CAD build for the part. Positions are in the model's coordinates, mm. A direction names the side the tool comes from. Coordinates: 2 decimals unless noted, no trailing zeros. Loops run counter-clockwise (first coordinate to the right, second up) from the corner with the lowest first, then second, coordinate; pieces in that order, holes last. Notation, with made-up numbers: (71, 69) - (103, 69) arc R24 ccw to (103, 99) - close; hole circle Ø6 at (87.5, 35.5). An arc over 180 degrees is marked (long way). Put each result on its own line as item: value.
```python
from build123d import *

# Parameters (mm, degrees)
SKETCH_1_W          = 28
SKETCH_1_H          = 45
EXTRUDE_1_DEPTH     = 2
SKETCH_2_W          = 25.5
SKETCH_2_H          = 40
EXTRUDE_2_DEPTH     = 13
EXTRUDE_3_DEPTH     = 11
SKETCH_4_W          = 20
SKETCH_4_H          = 24
CUT_EXTRUDE_1_DEPTH = 10


with BuildPart() as part:
    # 草图1 → 凸台-拉伸1 (new body)
    with BuildSketch(Plane.XY):
        Rectangle(SKETCH_1_W, SKETCH_1_H)
    extrude(amount=EXTRUDE_1_DEPTH)

    # 草图2 → 凸台-拉伸2 (add)
    with BuildSketch(Plane(origin=(0, 0, 0), x_dir=(-1, 0, 0), z_dir=(0, 0, -1))):
        Rectangle(SKETCH_2_W, SKETCH_2_H)
    extrude(amount=EXTRUDE_2_DEPTH)

    # 草图3 → 凸台-拉伸3 (add, symmetric)
    with BuildSketch(Plane(origin=(0, 0, 0), x_dir=(0, 0, -1), z_dir=(1, 0, 0))):
        Polygon((3, 20), (9, 20), (9, 30.5), (11, 30.5), (11, 33.5), (6, 38.5), (6, 30.5), (3, 30.5), align=None)
    extrude(amount=EXTRUDE_3_DEPTH, both=True)

    # 草图4 → 切除-拉伸1 (cut)
    with BuildSketch(Plane.XY.offset(2)):
        Rectangle(SKETCH_4_W, SKETCH_4_H)
    extrude(amount=-CUT_EXTRUDE_1_DEPTH, mode=Mode.SUBTRACT)


solid = part.part
```
Q1. Wall check: L1, parallel to Y at x = 4.25, z = -4.5; L2, parallel to X at y = 2, z = -7; L3, parallel to Y at x = 4.75, z = 0.75. Give the ranges that are in metal, low to high. Write a range as from..to.
Determined:
L1: -20..-12, 12..30.5
L2: -12.75..-10, 10..12.75
L3: -22.5..-12, 12..22.5
Q2. Pin check, flat tips, straight feed: pin 1 Ø1.6 at (x, z) = (3, -9.5) entering from -Y; pin 2 Ø4 at (y, z) = (1.5, -6.5) entering from +X; pin 3 Ø2 at (x, z) = (8, -5.5) entering from +Y. Stop position of each tip, or through.
Determined:
pin 1: y = -20
pin 2: x = 12.75
pin 3: y = 38.5
Q3. Slice it at C-C, the plane y = -1. Give the cut face in (x, z).
Determined:
outline: (-14, 0) - (-12.75, 0) - (-12.75, -13) - (12.75, -13) - (12.75, 0) - (14, 0) - (14, 2) - (10, 2) - (10, -8) - (-10, -8) - (-10, 2) - (-14, 2) - close
Q4. Mould opens along Z. For faces 1 (the flat face through (12.75, 0, -6)), 2 (the flat face through (0, 0, -13)), 3 (the flat face through (0, 25, -3)) say: +Z half, -Z half, draft (parallel to the pull), parting line (faces both ways), or undercut.
Determined:
face 1: draft
face 2: -Z half
face 3: undercut
Q5. Slice it at A-A, the plane z = -0.75. Give the cut face in (x, y), then the cut area to 3 significant figures.
Determined:
outline: (-12.75, -20) - (12.75, -20) - (12.75, 20) - (-12.75, 20) - close; hole (-10, -12) - (10, -12) - (10, 12) - (-10, 12) - close
area: 540 mm2
Q6. Slice it at B-B, the plane x = 7.75. Give the cut face in (y, z).
Determined:
outline: (-22.5, 0) - (-20, 0) - (-20, -13) - (20, -13) - (20, -9) - (30.5, -9) - (30.5, -11) - (33.5, -11) - (38.5, -6) - (30.5, -6) - (30.5, -3) - (20, -3) - (20, 0) - (22.5, 0) - (22.5, 2) - (12, 2) - (12, -8) - (-12, -8) - (-12, 2) - (-22.5, 2) - close
Q7. Slice it at D-D, the plane z = -7. Give the cut face in (x, y).
Determined:
outline: (-12.75, -20) - (12.75, -20) - (12.75, 20) - (11, 20) - (11, 37.5) - (-11, 37.5) - (-11, 20) - (-12.75, 20) - close; hole (-10, -12) - (10, -12) - (10, 12) - (-10, 12) - close
Q8. Tool access for faces 4 (the flat face through (-11, 27, -7)), 5 (the flat face through (0, 30.5, -5)), 6 (the flat face through (10, 0, -3)), 7 (the flat face through (0, 32, -11)): list every direction of +Z, -Z, +X, -X, +Y, -Y with a clear straight run to the whole face (end or side of a thin tool).
Determined:
face 4: -Z, -X, +Y
face 5: +Z, +X, -X, +Y
face 6: +Z
face 7: -Z, +X, -X, +Y
